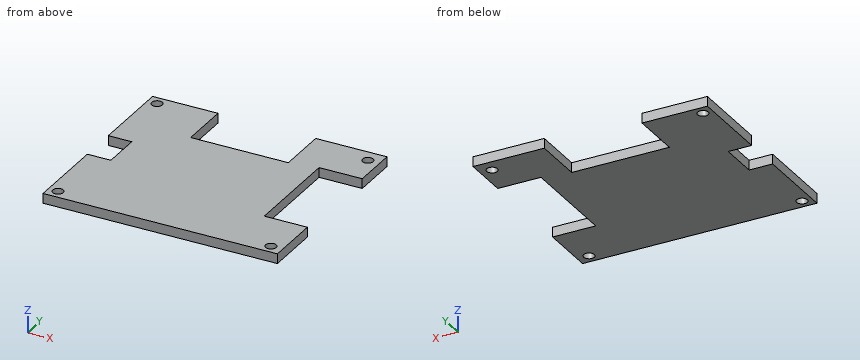
```python
from build123d import *

# Parameters (mm, degrees)
BOSS_EXTRUDE1_DEPTH       = 3.175
F_4_CLEARANCE_HOLE1_D     = 3.4544
F_4_CLEARANCE_HOLE1_DEPTH = 10.16
F_4_CLEARANCE_HOLE1_TIP   = 1.037806461


with BuildPart() as part:
    # Sketch2 → Boss-Extrude1 (new body)
    with BuildSketch(Plane.XY):
        Polygon((-38.1, 33.02), (-16.8275, 33.02), (-16.8275, 16.51), (14.9225, 16.51), (14.9225, 33.02), (38.1, 33.02), (38.1, 18.1011502), (24.060772257, 18.1011502), (24.060772257, -14.926152342), (38.1, -14.926152342), (38.1, -33.02), (-38.1, -33.02), (-38.1, -6.305887107), (-30.445430268, -6.305887107), (-30.445430268, 6.305887107), (-38.1, 6.305887107), align=None)
    extrude(amount=BOSS_EXTRUDE1_DEPTH)

    # #4 Clearance Hole1
    with Locations(Plane.XY.offset(3.175)):
        with Locations((-34.925, 29.845), (34.29, 28.575), (-34.925, -29.845), (34.29, -29.845)):
            Hole(F_4_CLEARANCE_HOLE1_D / 2, depth=F_4_CLEARANCE_HOLE1_DEPTH)
            with Locations((0, 0, -(F_4_CLEARANCE_HOLE1_DEPTH + F_4_CLEARANCE_HOLE1_TIP / 2))):  # 118° drill point
                Cone(0, F_4_CLEARANCE_HOLE1_D / 2, F_4_CLEARANCE_HOLE1_TIP, mode=Mode.SUBTRACT)


solid = part.part
```
Build history of the part. All positions in model axes, mm. Round coordinates to 2 decimals unless told otherwise and drop trailing zeros. Order: outer loops, then holes, each group sorted by start corner. A loop starts at its lowest first (then second) coordinate and runs counter-clockwise, first axis right, second up. Notation, with made-up numbers: (21, 43) - (30, 43) arc R29 cw to (30, 63) - close; hole circle Ø1 at (82, 17.5). An arc over 180 degrees is marked (long way). Use a Markdown table: item, result.
1) Saw through at C-C on z = 2.2. Write the cut outline in (x, y) (1 decimal).
Recorded:
| item | result |
|---|---|
| outline | (-38.1, -33) - (38.1, -33) - (38.1, -14.9) - (24.1, -14.9) - (24.1, 18.1) - (38.1, 18.1) - (38.1, 33) - (14.9, 33) - (14.9, 16.5) - (-16.8, 16.5) - (-16.8, 33) - (-38.1, 33) - (-38.1, 6.3) - (-30.4, 6.3) - (-30.4, -6.3) - (-38.1, -6.3) - close; hole circle Ø3.5 at (-34.9, -29.8); hole circle Ø3.5 at (-34.9, 29.8); hole circle Ø3.5 at (34.3, -29.8); hole circle Ø3.5 at (34.3, 28.6) |
2) Flat gauge pins, fed straight in: pin 1 Ø1.5 at (x, y) = (-9, -24) entering from -Z; pin 2 Ø1.6 at (y, z) = (0.5, 2) entering from -X; pin 3 Ø1 at (x, z) = (1, 1.5) entering from +Y. Where does each tip first touch, or does it go through?
Recorded:
| item | result |
|---|---|
| pin 1 | stops at z = 0 |
| pin 2 | stops at x = -30.45 |
| pin 3 | stops at y = 16.51 |
3) Saw through at D-D on x = 11. Write the cut outline in (y, z) (3 decimals), and give its area (3 significant figures).
Recorded:
| item | result |
|---|---|
| outline | (-33.02, 0) - (16.51, 0) - (16.51, 3.175) - (-33.02, 3.175) - close |
| area | 157 mm² |
4) Saw through at B-B on y = 23. Write the cut outline in (x, z) (1 decimal), and give its area (3 significant figures).
Recorded:
| item | result |
|---|---|
| outline | (-38.1, 0) - (-16.8, 0) - (-16.8, 3.2) - (-38.1, 3.2) - close; (14.9, 0) - (38.1, 0) - (38.1, 3.2) - (14.9, 3.2) - close |
| area | 141 mm² |
5) Saw through at A-A on x = 34.29. Write the cut outline in (y, z) (3 decimals), and give its area (3 significant figures).
Recorded:
| item | result |
|---|---|
| outline | (-33.02, 0) - (-31.572, 0) - (-31.572, 3.175) - (-33.02, 3.175) - close; (-28.118, 0) - (-14.926, 0) - (-14.926, 3.175) - (-28.118, 3.175) - close; (18.101, 0) - (26.848, 0) - (26.848, 3.175) - (18.101, 3.175) - close; (30.302, 0) - (33.02, 0) - (33.02, 3.175) - (30.302, 3.175) - close |
| area | 82.9 mm² |
6) Wall check: L1, parallel to Y at x = 34.29, z = 1.05; L2, parallel to Y at x = 31, z = 0.9; L3, parallel to X at y = 24, z = 1.5. Give the ranges that are in metal, low to high.
Recorded:
| item | result |
|---|---|
| L1 | y = -33.02 to -31.57, -28.12 to -14.93, 18.1 to 26.85, 30.3 to 33.02 |
| L2 | y = -33.02 to -14.93, 18.1 to 33.02 |
| L3 | x = -38.1 to -16.83, 14.92 to 38.1 |
